Source: CAD feature listing. Evaluate the final solid. Frame: model axes, mm. Face numbers are marked on the shaded views. A direction names the side the tool comes from. Give positions to 0.01 mm unless a question says otherwise; leave off trailing zeros. Loops run counter-clockwise (first coordinate to the right, second up) from the corner with the lowest first, then second, coordinate; pieces in that order, holes last. Notation, with made-up numbers: M 49,-7 L 60,-7 A20 ccw 60,6 Z; hole C -32.5,57 d6. An arc over 180 degrees is marked long. Answer in a Markdown table with one row per item.
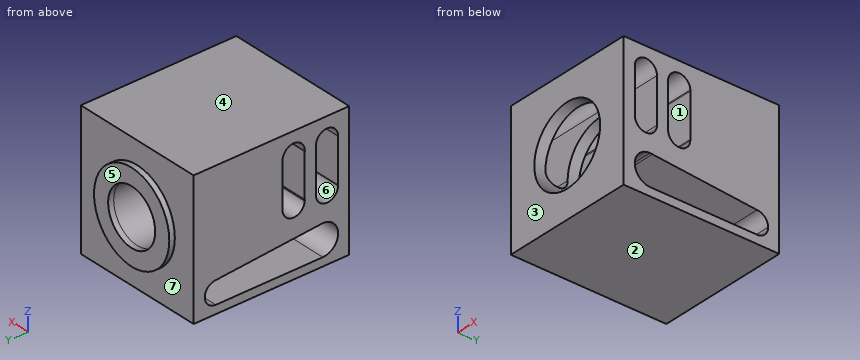
```python
from build123d import *

# Parameters (mm, degrees)
F0_W      = 30.48
F0_H      = 30.48
F1_DEPTH  = 35.56
F3_DEPTH  = 38.1
F5_DEPTH  = 38.1
F6_R      = 8.89
F7_DEPTH  = 22.86
F8_R      = 10.16
F9_DEPTH  = 1.27
F10_R     = 6.35
F11_DEPTH = 38.1
F12_R     = 6.35
F13_DEPTH = 25.4


with BuildPart() as f1:
    # F0 (on Front) → F1 (new body)
    with BuildSketch(Plane.XZ):
        Rectangle(F0_W, F0_H)
    extrude(amount=F1_DEPTH)

    # F2 (on face) → F3 (cut)
    with BuildSketch(Plane(origin=(-15.24, 0, 0), x_dir=(0, -1, 0), z_dir=(-1, 0, 0))):
        with BuildLine():
            ThreePointArc((33.017656, 10.050903), (33.019414, 10.105439), (33.02, 10.16))
            ThreePointArc((33.02, 10.16), (30.48, 12.7), (27.94, 10.16))
            ThreePointArc((27.94, 10.16), (30.425439, 7.620586), (33.017656, 10.050903))
        make_face()
        with BuildLine():
            ThreePointArc((33.017656, 10.050903), (30.425439, 7.620586), (27.94, 10.16))
            Line((27.94, 10.16), (27.94, 0))
            ThreePointArc((27.94, 0), (30.425439, 2.539414), (33.017656, 0.109097))
            Line((33.017656, 0.109097), (33.017656, 10.050903))
        make_face()
        with BuildLine():
            ThreePointArc((33.017656, 0.109097), (30.425439, 2.539414), (27.94, 0))
            ThreePointArc((27.94, 0), (30.425439, -2.539414), (33.017656, -0.109097))
            Line((33.017656, -0.109097), (33.017656, 0.109097))
        make_face()
        with BuildLine():
            ThreePointArc((33.02, 0), (33.019414, 0.054561), (33.017656, 0.109097))
            Line((33.017656, 0.109097), (33.017656, -0.109097))
            ThreePointArc((33.017656, -0.109097), (33.019414, -0.054561), (33.02, 0))
        make_face()
        with BuildLine():
            ThreePointArc((25.391599, 9.953588), (25.397899, 10.056709), (25.4, 10.16))
            ThreePointArc((25.4, 10.16), (22.926198, 12.699137), (20.323451, 10.292352))
            Line((20.323451, 10.292352), (20.323451, 10.027648))
            ThreePointArc((20.323451, 10.027648), (22.822887, 7.620271), (25.391599, 9.953588))
        make_face()
        with BuildLine():
            Line((20.323451, 10.027648), (20.323451, 10.292352))
            ThreePointArc((20.323451, 10.292352), (20.32, 10.16), (20.323451, 10.027648))
        make_face()
        with BuildLine():
            Line((25.391599, 0.206412), (25.391599, 9.953588))
            ThreePointArc((25.391599, 9.953588), (22.822887, 7.620271), (20.323451, 10.027648))
            Line((20.323451, 10.027648), (20.323451, 0.132352))
            ThreePointArc((20.323451, 0.132352), (22.822887, 2.539729), (25.391599, 0.206412))
        make_face()
        with BuildLine():
            Line((25.391599, -0.206412), (25.391599, 0.206412))
            ThreePointArc((25.391599, 0.206412), (22.822887, 2.539729), (20.323451, 0.132352))
            Line((20.323451, 0.132352), (20.323451, -0.132352))
            ThreePointArc((20.323451, -0.132352), (22.822887, -2.539729), (25.391599, -0.206412))
        make_face()
        with BuildLine():
            ThreePointArc((25.4, 0), (25.397899, 0.103291), (25.391599, 0.206412))
            Line((25.391599, 0.206412), (25.391599, -0.206412))
            ThreePointArc((25.391599, -0.206412), (25.397899, -0.103291), (25.4, 0))
        make_face()
        with BuildLine():
            Line((20.323451, -0.132352), (20.323451, 0.132352))
            ThreePointArc((20.323451, 0.132352), (20.32, 0), (20.323451, -0.132352))
        make_face()
    extrude(amount=-F3_DEPTH, mode=Mode.SUBTRACT)

    # F4 (on face) → F5 (cut)
    with BuildSketch(Plane.YZ.offset(15.24)):
        with BuildLine():
            Line((-28.986499, -6.392156), (-29.5275, -6.35))
            ThreePointArc((-29.5275, -6.35), (-33.02, -9.8425), (-29.5275, -13.335))
            ThreePointArc((-29.5275, -13.335), (-27.05793, -12.31207), (-26.035, -9.8425))
            ThreePointArc((-26.035, -9.8425), (-26.873541, -7.572246), (-28.986499, -6.392156))
        make_face()
        with BuildLine():
            ThreePointArc((-28.986499, -6.392156), (-29.25618, -6.360555), (-29.5275, -6.35))
            Line((-29.5275, -6.35), (-28.986499, -6.392156))
        make_face()
        with BuildLine():
            ThreePointArc((-26.035, -9.8425), (-27.05793, -12.31207), (-29.5275, -13.335))
            Line((-29.5275, -13.335), (-5.08, -13.335))
            ThreePointArc((-5.08, -13.335), (-7.62, -10.795), (-5.08, -8.255))
            Line((-5.08, -8.255), (-28.986499, -6.392156))
            ThreePointArc((-28.986499, -6.392156), (-26.873541, -7.572246), (-26.035, -9.8425))
        make_face()
        with BuildLine():
            ThreePointArc((-5.08, -8.255), (-7.62, -10.795), (-5.08, -13.335))
            ThreePointArc((-5.08, -13.335), (-3.283949, -12.591051), (-2.54, -10.795))
            ThreePointArc((-2.54, -10.795), (-3.283949, -8.998949), (-5.08, -8.255))
        make_face()
    extrude(amount=-F5_DEPTH, mode=Mode.SUBTRACT)

    # F6 (on face) → F7 (cut)
    with BuildSketch(Plane.XZ.offset(35.56)):
        Circle(F6_R)
    extrude(amount=-F7_DEPTH, mode=Mode.SUBTRACT)

    # F8 (on face) → F9 (join)
    with BuildSketch(Plane(origin=(0, 0, 0), x_dir=(-1, 0, 0), z_dir=(0, 1, 0))):
        Circle(F8_R)
    extrude(amount=F9_DEPTH)

    # F10 (on face) → F11 (cut)
    with BuildSketch(Plane.XZ):
        Circle(F10_R)
    extrude(amount=-F11_DEPTH, mode=Mode.SUBTRACT)

    # F12 (on face) → F13 (cut)
    with BuildSketch(Plane(origin=(0, 0, 0), x_dir=(-1, 0, 0), z_dir=(0, 1, 0))):
        Circle(F12_R)
    extrude(amount=-F13_DEPTH, mode=Mode.SUBTRACT)


solid = f1.part
```
Q1. Ray query, probe 1 along Y at (x, z) = (-7.5, 8.5); probe 2 along Z at (x, y) = (-5.5, -9.5) (3 decimals); probe 3 along Y at (x, z) = (13, -1). Return the intervals inside material, ascending. Write a range as from..to.
Values follow:
| item | result |
|---|---|
| probe 1 | -35.56..-33.02, -27.94..-25.39, -20.32..0 |
| probe 2 | -15.24..-13.335, -7.911..-3.174, 3.174..15.24 |
| probe 3 | -35.56..-32.81, -28.15..-25.19, -20.53..0 |
Q2. Mould query, pull axis Z, two halves, no side actions, for the marked faces 1, 2, 3 and 4. Classes: +Z half, -Z half, draft (parallel to the pull), parting line (faces both ways), or undercut.
Values follow:
| item | result |
|---|---|
| face 1 | undercut |
| face 2 | -Z half |
| face 3 | draft |
| face 4 | +Z half |
Q3. Section query D-D (y = -31). Output: boundary loops of the cut face in (x, z), plus the area to 3 significant figures.
Values follow:
| item | result |
|---|---|
| outline | M -15.24,-15.24 L 15.24,-15.24 L 15.24,-13.01 L -15.24,-13.01 Z; M -15.24,-6.68 L -5.87,-6.68 A8.89 cw -8.54,-2.49 L -15.24,-2.49 Z; M -15.24,12.65 L 15.24,12.65 L 15.24,15.24 L -15.24,15.24 Z; M 5.87,-6.68 L 15.24,-6.68 L 15.24,-2.49 L 8.54,-2.49 A8.89 cw Z |
| area | 212 mm^2 |
Q4. Contact query for flat-ended pins moving along their axis: pin 1 Ø4 at (x, z) = (10.5, -10) entering from +Y; pin 2 Ø3 at (x, z) = (2.5, 4.5) entering from -Y. Output: stop coordinate, or through.
Values follow:
| item | result |
|---|---|
| pin 1 | y = 0 |
| pin 2 | y = -12.7 |
Q5. Section query A-A (y = -9.5). Output: boundary loops of the cut face in (x, z) (3 decimals), plus the area to 3 significant figures.
Values follow:
| item | result |
|---|---|
| outline | M -15.24,-15.24 L 15.24,-15.24 L 15.24,-13.335 L -15.24,-13.335 Z; M -15.24,-7.911 L 15.24,-7.911 L 15.24,15.24 L -15.24,15.24 Z; hole C 0,0 d12.7 |
| area | 637 mm^2 |
Q6. Reachability of the marked faces 5, 6 and 7 from +Z, -Z, +X, -X, +Y, -Y: full face, straight path, thin tool, end or side. Return the list, or none.
Values follow:
| item | result |
|---|---|
| face 5 | +Z, -Z, +X, -X, +Y |
| face 6 | +X, -X |
| face 7 | +Y |
Q7. Section query B-B (z = -2). Give the number of separate pieces and of enclosed holes in the cut face, plus the area to 3 significant figures.
Values follow:
| item | result |
|---|---|
| separate pieces | 6 |
| enclosed holes | 0 |
| area | 462 mm^2 |
